Read the model definition and answer for the solid it produces. Units are mm, in the model's axes. Face numbers are marked on the shaded views. A direction names the side the tool comes from. Round coordinates to 2 decimals unless told otherwise and drop trailing zeros. Write each loop counter-clockwise with the first axis right and the second up, starting at its lowest first coordinate (ties: lowest second). Pieces come first, ordered by that corner, then holes.
Autodesk Inventor part; units mm, degrees
ref_plane "YZ Plane" through (0, 0, 0) normal (1, 0, 0) x (0, 1, 0)
ref_plane "XZ Plane" through (0, 0, 0) normal (0, 1, 0) x (-1, 0, 0)
ref_plane "XY Plane" through (0, 0, 0) normal (0, 0, 1) x (1, 0, 0)
sketch "Boceto1" plane through (0, 0, 0) normal (0, 0, 1) x (1, 0, 0)
  circle A0 centre (0, 0) radius 12.5
  dimension "d0" = 25
extrude "Extrusión1" add sketch "Boceto1" along normal blind 40
sketch "Boceto2" plane through (0, 0, 40) normal (0, 0, 1) x (1, 0, 0)
  circle A0 centre (0, 0) radius 12.5
  line L0 (0, 12.5) -> (12.5, 0)
  line L1 (0, -12.5) -> (12.5, 0)
  line L2 (0, 12.5) -> (-12.5, 0)
  line L3 (-12.5, 0) -> (0, -12.5)
extrude "Extrusión2" add sketch "Boceto2" along normal blind 10 contours L1 L3 L2 L0
properties part number "ejeM"
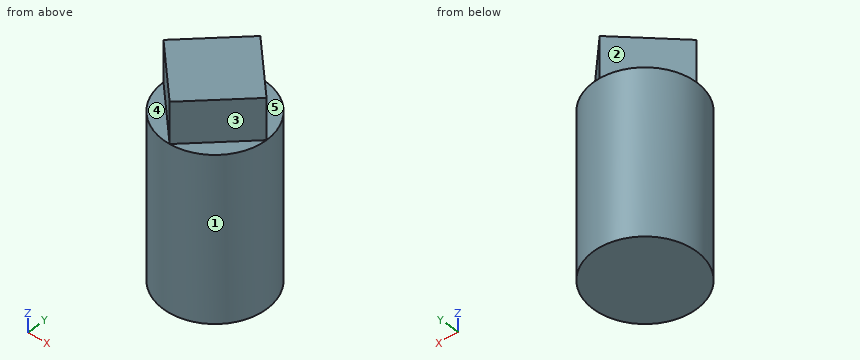
Q1. Section D-D (z = 46.5) is taken. Determine the outline of the cut face in (x, y).
Verdict:
outline: (-12.5, 0) - (0, -12.5) - (12.5, 0) - (0, 12.5) - close
Q2. Straight lines are drawn through the part: probe 1 along Z at (x, y) = (8.25, 8.25); probe 2 along Y at (x, z) = (-0.25, 32.5); probe 3 along Y at (x, z) = (-6, 30.5). For each, find the intervals that lie inside material, in ascending order.
Verdict:
probe 1: z = 0 to 40
probe 2: y = -12.5 to 12.5
probe 3: y = -10.97 to 10.97
Q3. Section C-C (z = 22.5) is taken. Determine the outline of the cut face in (x, y).
Verdict:
outline: circle Ø25 at (0, 0)
Q4. Section B-B (x = 9) is taken. Determine the outline of the cut face in (y, z), then the cut area to 3 significant figures.
Verdict:
outline: (-8.67, 0) - (8.67, 0) - (8.67, 40) - (3.5, 40) - (3.5, 50) - (-3.5, 50) - (-3.5, 40) - (-8.67, 40) - close
area: 764 mm2
Q5. Flat-ended cylindrical pins translate along their axes: pin 1 Ø12 at (x, z) = (9.5, 16) entering from -Y; pin 2 Ø6 at (y, z) = (6, 38) entering from +X; pin 3 Ø1 at (y, z) = (2, 5.5) entering from -X. Find the tip coordinate at first contact, or state that the pin passes through.
Verdict:
pin 1: stops at y = -12
pin 2: stops at x = 12.13
pin 3: stops at x = -12.41
Q6. Section A-A (y = 10.75) is taken. Determine the outline of the cut face in (x, z).
Verdict:
outline: (-6.38, 0) - (6.38, 0) - (6.38, 40) - (1.75, 40) - (1.75, 50) - (-1.75, 50) - (-1.75, 40) - (-6.38, 40) - close
Q7. Which of the six approach directions +Z, -Z, +X, -X, +Y, -Y give full straight-line access (tool end or side, diameter ignored) to the marked faces 1, 2, 3, 4 and 5?
Verdict:
face 1: +Z, -Z
face 2: +Z, -X, +Y
face 3: +Z, +X, -Y
face 4: +Z, -X, -Y
face 5: +Z, +X, +Y
